The figure shows three views and two pictorial views of one solid part (mm, origin at its lowest corner). Answer the questions. A direction names the side the tool comes from. Round coordinates to 2 decimals unless told otherwise and drop trailing zeros. Order: outer loops, then holes, each group sorted by start corner. A loop starts at its lowest first (then second) coordinate and runs counter-clockwise, first axis right, second up. Notation, with made-up numbers: M 76.25,-25 L 91.25,-25 A14 cw 91.25,-7 Z; hole C 35.5,-38 d3. An arc over 180 degrees is marked long. Answer as CSV lines item,"result".
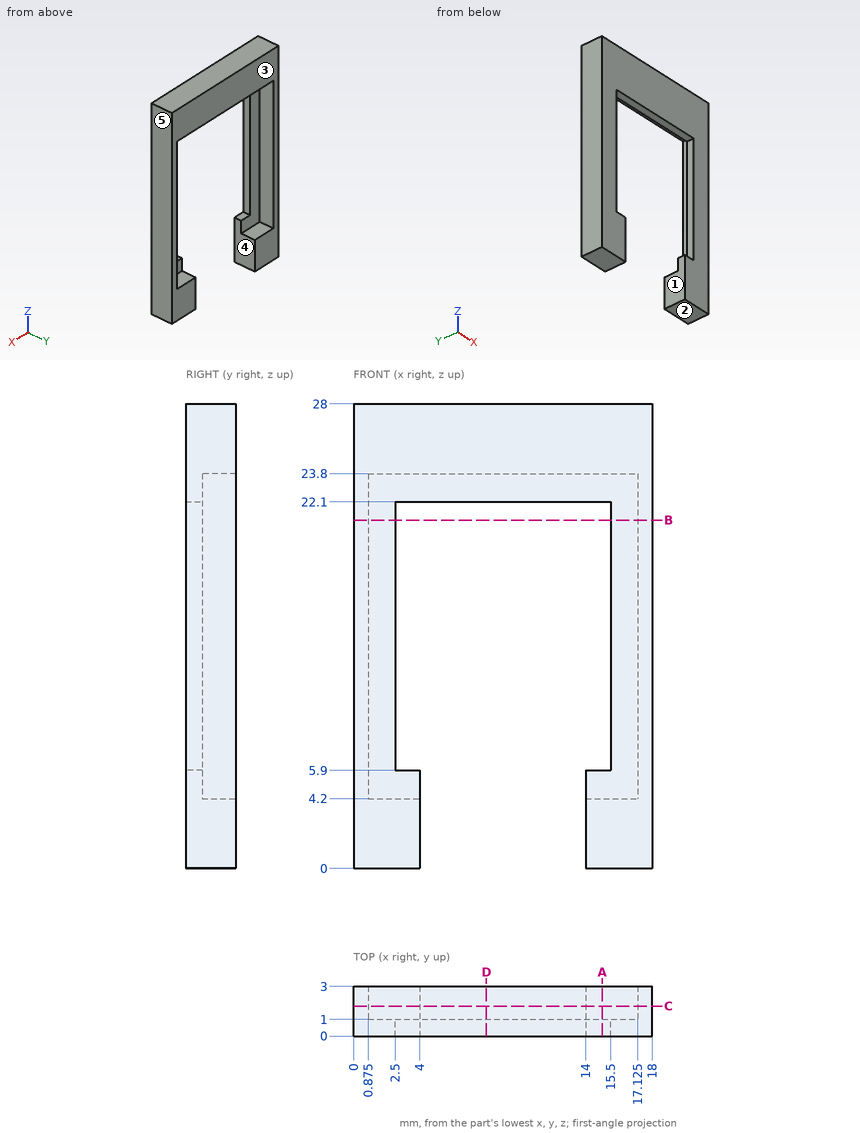
Item 1: Flat-ended cylindrical pins translate along their axes: pin 1 (10 mm diameter, centred on x = 11.5, z = 12, fed in from +Y); pin 2 (0.9 mm diameter, centred on y = 1, z = 4.5, fed in from -X); pin 3 (0.8 mm diameter, centred on x = 7, y = 0.5, fed in from -Z); pin 4 (1 mm diameter, centred on x = 10.5, y = 2, fed in from -Z). Find the tip coordinate at first contact, or state that the pin passes through.
Ans:
pin 1,"y = 1"
pin 2,"x = 0"
pin 3,"z = 22.1"
pin 4,"z = 23.8"
Item 2: A cutting plane is placed at D-D, the plane x = 8. Determine the outline of the cut face in (y, z), and give its area (3 significant figures).
Ans:
outline,"M 0,22.1 L 1,22.1 L 1,23.8 L 3,23.8 L 3,28 L 0,28 Z"
area,"14.3 mm2"
Item 3: A tool of negligible diameter and unlimited length cuts with its end or side. For the marked faces 1 and 2, from which of +Z, -Z, +X, -X, +Y, -Y can it reach the whole face along a straight path? Write none if from no direction.
Ans:
face 1,"-Z, +Y, -Y"
face 2,"-Z, +X, -X, +Y, -Y"
Item 4: A cutting plane is placed at A-A, the plane x = 15. Determine the outline of the cut face in (y, z).
Ans:
outline,"M 0,0 L 3,0 L 3,4.2 L 1,4.2 L 1,5.9 L 0,5.9 Z; M 0,22.1 L 1,22.1 L 1,23.8 L 3,23.8 L 3,28 L 0,28 Z"
Item 5: Determine the mould class of the marked faces 3, 4 and 5 for opening direction X: +X half, -X half, draft (parallel to the pull), parting line (faces both ways), or undercut.
Ans:
face 3,"draft"
face 4,"undercut"
face 5,"+X half"
Item 6: Find the intervals of material crossed by probe 1 along X at (y, z) = (1.4, 21.75) (3 decimals); probe 2 along Z at (x, y) = (14.25, 0.95); probe 3 along X at (y, z) = (0.5, 18.25), in increasing order. Write a range as [from, to].
Ans:
probe 1,"[0, 0.875], [17.125, 18]"
probe 2,"[0, 5.9], [22.1, 28]"
probe 3,"[0, 2.5], [15.5, 18]"
Item 7: A cutting plane is placed at B-B, the plane z = 21. Determine the outline of the cut face in (x, y) (3 decimals), and give its area (3 significant figures).
Ans:
outline,"M 0,0 L 2.5,0 L 2.5,1 L 0.875,1 L 0.875,3 L 0,3 Z; M 15.5,0 L 18,0 L 18,3 L 17.125,3 L 17.125,1 L 15.5,1 Z"
area,"8.50 mm2"
Item 8: A cutting plane is placed at C-C, the plane y = 1.8. Determine the outline of the cut face in (x, z) (3 decimals).
Ans:
outline,"M 0,0 L 4,0 L 4,4.2 L 0.875,4.2 L 0.875,23.8 L 17.125,23.8 L 17.125,4.2 L 14,4.2 L 14,0 L 18,0 L 18,28 L 0,28 Z"
